```python
from build123d import *

# Parameters (mm, degrees)
SKETCH3_W           = 160
SKETCH3_H           = 56
BOSS_EXTRUDE1_DEPTH = 3
SKETCH4_W           = 3
SKETCH4_H           = 10
SKETCH4_W_2         = 35
SKETCH4_H_2         = 3
CUT_EXTRUDE1_DEPTH  = 85.811555816


with BuildPart() as part:
    # Sketch3 → Boss-Extrude1 (new body)
    with BuildSketch(Plane(origin=(0, 0, 0), x_dir=(1, 0, 0), z_dir=(0, 1, 0))):
        Rectangle(SKETCH3_W, SKETCH3_H)
    extrude(amount=BOSS_EXTRUDE1_DEPTH)

    # Sketch4 → Cut-Extrude1 (cut, through all)
    with BuildSketch(Plane(origin=(0, 3, 0), x_dir=(1, 0, 0), z_dir=(0, 1, 0))):
        with Locations((-78.5, 12.5)):
            Rectangle(SKETCH4_W, SKETCH4_H)
        Polygon((-35, 28), (-35, 25), (-1.5, 25), (-1.5, 20.5), (-3, 20.5), (-3, 18), (3, 18), (3, 20.5), (1.5, 20.5), (1.5, 25), (35, 25), (35, 28), align=None)
        with Locations((-62.5, 26.5)):
            Rectangle(SKETCH4_W_2, SKETCH4_H_2)
        with Locations((62.5, 26.5)):
            Rectangle(SKETCH4_W_2, SKETCH4_H_2)
        with Locations((78.5, 12.5)):
            Rectangle(SKETCH4_W, SKETCH4_H)
        with Locations((78.5, -12.5)):
            Rectangle(SKETCH4_W, SKETCH4_H)
        with Locations((62.5, -26.5)):
            Rectangle(SKETCH4_W_2, SKETCH4_H_2)
        Polygon((35, -28), (-35, -28), (-35, -25), (-1.5, -25), (-1.5, -20.5), (-3, -20.5), (-3, -18), (3, -18), (3, -20.5), (1.5, -20.5), (1.5, -25), (35, -25), align=None)
        with Locations((-62.5, -26.5)):
            Rectangle(SKETCH4_W_2, SKETCH4_H_2)
        with Locations((-78.5, -12.5)):
            Rectangle(SKETCH4_W, SKETCH4_H)
    extrude(amount=-CUT_EXTRUDE1_DEPTH, mode=Mode.SUBTRACT)


solid = part.part
```
The listing builds one solid part. Answer for the finished solid, in the listing's coordinates (mm). A direction names the side the tool comes from. Give positions to 0.01 mm unless a question says otherwise; leave off trailing zeros. Order: outer loops, then holes, each group sorted by start corner. A loop starts at its lowest first (then second) coordinate and runs counter-clockwise, first axis right, second up.
1) Determine the mould class of faces 6 (the face through (78, 2, 17.5)), 7 (the face through (35, 2, -26)), 8 (the face through (-77, 2, -12)) for opening direction X: pulls with the +X half, pulls with the -X half, needs draft (parallel to the pull), parting line crosses it, or undercut.
Reported:
face 6: needs draft
face 7: undercut
face 8: pulls with the -X half
2) For faces 1 (the face through (35, 2, 26)), 2 (the face through (62, 2, 25)), 3 (the face through (45, 2, -26)), 4 (the face through (0, 2, 18)), 5 (the face through (-45, 2, 27)), determine the directions among +Z, -Z, +X, -X, +Y, -Y from which every point of the face is accessible in a straight line to the end or side of a thin tool.
Reported:
face 1: +Z, +Y, -Y
face 2: +Z, +X, +Y, -Y
face 3: -Z, +X, +Y, -Y
face 4: +Y, -Y
face 5: +Z, -X, +Y, -Y
3) Find section B-B on x = -22. Write down the section's boundary in (y, z).
Reported:
outline: (0, -25) - (3, -25) - (3, 25) - (0, 25) - close
4) Find section C-C on z = -14. Write down the section's boundary in (x, y), then the cut area to 3 significant figures.
Reported:
outline: (-77, 0) - (77, 0) - (77, 3) - (-77, 3) - close
area: 462 mm2
5) Find section A-A on z = -23. Write down the section's boundary in (x, y), then the cut area to 3 significant figures.
Reported:
outline: (-80, 0) - (-1.5, 0) - (-1.5, 3) - (-80, 3) - close; (1.5, 0) - (80, 0) - (80, 3) - (1.5, 3) - close
area: 471 mm2
6) Consider line 1 along X through (y, z) = (1.3, 19.5); line 2 along X through (y, z) = (1.15, 25.5); line 3 along Z through (x, y) = (17, 1.45). Determine where each line is inside the solid, lowest interval first.
Reported:
line 1: x = -80 to -3, 3 to 80
line 2: x = -45 to -35, 35 to 45
line 3: z = -25 to 25
7) Given P1, Ø0.9, axis at x = -78.5, y = 2, coming from the +Z side; P2, Ø1.5, axis at y = 1, z = 26.5, coming from the +X side; P3, Ø1.5, axis at x = 62, y = 1, coming from the -Z side, each flat-ended and moving along its own axis, determine where each tip first touches the part or whether it passes through.
Reported:
P1: stops at z = 25
P2: stops at x = 45
P3: stops at z = -25
